Geometry check sheet. Reference: the model listing, model coordinates, mm. A direction names the side the tool comes from. Round coordinates to 2 decimals unless told otherwise and drop trailing zeros. Write each loop counter-clockwise with the first axis right and the second up, starting at its lowest first coordinate (ties: lowest second). Pieces come first, ordered by that corner, then holes. Notation, with made-up numbers: (31.5, -4) - (71.5, -4) arc R5 ccw to (71.5, 2) - close; hole circle Ø8 at (0, -20). An arc over 180 degrees is marked (long way). One line per question, with ' | ' between items. Start each with the question number.
from build123d import *

# Parameters (mm, degrees)
SKETCH1_R           = 2
BOSS_EXTRUDE1_DEPTH = 2
SKETCH2_R           = 4
BOSS_EXTRUDE2_DEPTH = 3
CUT_EXTRUDE1_DEPTH  = 2


with BuildPart() as part:
    # Sketch1 → Boss-Extrude1 (new body)
    with BuildSketch(Plane(origin=(0, 0, 0), x_dir=(1, 0, 0), z_dir=(0, 1, 0))):
        with Locations(Location((0, 0, 0), (0, 0, 270))):
            Circle(SKETCH1_R)
    extrude(amount=BOSS_EXTRUDE1_DEPTH)

    # Sketch2 → Boss-Extrude2 (add)
    with BuildSketch(Plane(origin=(0, 2, 0), x_dir=(1, 0, 0), z_dir=(0, 1, 0))):
        with Locations(Location((0, 0, 0), (0, 0, 270))):
            Circle(SKETCH2_R)
    extrude(amount=BOSS_EXTRUDE2_DEPTH)

    # Sketch3 → Cut-Extrude1 (cut)
    with BuildSketch(Plane(origin=(0, 5, 0), x_dir=(1, 0, 0), z_dir=(0, 1, 0))):
        Polygon((3.19667155, 0), (1.598335775, 2.76839877), (-1.598335775, 2.76839877), (-3.19667155, 0), (-1.598335775, -2.76839877), (1.598335775, -2.76839877), align=None)
    extrude(amount=-CUT_EXTRUDE1_DEPTH, mode=Mode.SUBTRACT)


solid = part.part
Q1. Section check A-A, the plane y = 3.3. Record the cut outline in (x, z), then the cut area to 3 significant figures.
Q2. Section check B-B, the plane x = 0. Record the cut outline in (y, z).
Q3. Section check C-C, the plane y = 1.35. Record the cut outline in (x, z).
Q4. Draft check along X on faces 4 (the flat face through (0, 0, 0)), 5 (the cylindrical face through (-3.905, 3.479, -0.867)), 6 (the flat face through (2.39, 4.01, 1.4)). Enter one of: pulls with the +X half, pulls with the -X half, needs draft (parallel to the pull), parting line crosses it, or undercut.
Q5. Set-up check for faces 1 (the flat face through (0, 4, -2.768)), 2 (the flat face through (3, 5, 1)), 3 (the cylindrical face through (-2, 1, 0)): record each of +Z, -Z, +X, -X, +Y, -Y from which the full face is reachable in a straight line by a thin tool's end or side.
Q6. Go/stop test with flat-tipped pins: P1, Ø1.5, axis at x = -3, z = -2, coming from the -Y side; P2, Ø3, axis at x = 2, y = 2.5, coming from the +Z side. Record where each tip stops, or that it passes through.
Q7. Thickness scan on line 1 (Y direction, x = -2.75, z = -2.5); line 2 (Y direction, x = -2.5, z = 1); line 3 (Z direction, x = 1.5, y = 3.2). Record the ranges inside material, lowest first.
Q8. Section check D-D, the plane z = 2.25. Record the cut outline in (x, y), then the cut area to 3 significant figures.
Result sheet:
1) outline: circle Ø8 at (0, 0); hole (-3.2, 0) - (-1.6, -2.77) - (1.6, -2.77) - (3.2, 0) - (1.6, 2.77) - (-1.6, 2.77) - close | area: 23.7 mm²
2) outline: (0, -2) - (2, -2) - (2, -4) - (5, -4) - (5, -2.77) - (3, -2.77) - (3, 2.77) - (5, 2.77) - (5, 4) - (2, 4) - (2, 2) - (0, 2) - close
3) outline: circle Ø4 at (0, 0)
4) face 4: needs draft | face 5: parting line crosses it | face 6: undercut
5) face 1: +Y | face 2: +Z, -Z, +X, -X, +Y | face 3: -Y
6) P1: y = 2 | P2: z = 3.97
7) line 1: 2 to 5 | line 2: 2 to 3 | line 3: -3.71 to -2.77, 2.77 to 3.71
8) outline: (-3.31, 2) - (3.31, 2) - (3.31, 5) - (1.9, 5) - (1.9, 3) - (-1.9, 3) - (-1.9, 5) - (-3.31, 5) - close | area: 12.3 mm²
